Model file for the job. Use its own axes, mm. Coordinates: 2 decimals unless noted, no trailing zeros. Write each loop counter-clockwise with the first axis right and the second up, starting at its lowest first coordinate (ties: lowest second). Pieces come first, ordered by that corner, then holes. Notation, with made-up numbers: (3, 11) - (53, 11) arc R8 cw to (53, 20) - close; hole circle Ø11 at (7.25, 7.25). An arc over 180 degrees is marked (long way). Put each result on its own line as item: value. Start each with the question number.
1. Drill centre lines: L1, parallel to X at y = 29, z = 1.8; L2, parallel to X at y = 3, z = 4.05 (3 decimals); L3, parallel to Y at x = -29, z = 0.4. Where is each one in solid material? Low to high. Write a range as from..to.
2. Drop flat-ended pins along their axis: P1, Ø22, axis at x = 0, y = 32.78, coming from the +Z side; P2, Ø10, axis at x = 32.78, y = 0, coming from the +Z side; P3, Ø2, axis at x = -40, z = 3, coming from the +Y side; P4, Ø1, axis at x = -11.5, z = 1.5, coming from the -Y side (3 decimals). Give the stop position or say it passes through.
3. Saw through at A-A, the plane z = 3.2. Give the number of separate pieces and of enclosed holes in the cut face, plus the area to 3 significant figures.
4. Saw through at B-B, the plane x = 0. Write the cut outline in (y, z), plus the area to 3 significant figures.
```python
from build123d import *

# Parameters (mm, degrees)
F0_R     = 50
F0_R_2   = 8.5
F1_DEPTH = 5
F2_R     = 1


with BuildPart() as f1:
    # F0 (on Top) → F1 (new body)
    with BuildSketch(Plane.XY):
        Circle(F0_R)
        with Locations((-23.180378, -23.180378)):
            Circle(F0_R_2, mode=Mode.SUBTRACT)
        with Locations((0, -32.782005)):
            Circle(F0_R_2, mode=Mode.SUBTRACT)
        with Locations((23.180378, -23.180378)):
            Circle(F0_R_2, mode=Mode.SUBTRACT)
        with Locations((-32.782005, 0)):
            Circle(F0_R_2, mode=Mode.SUBTRACT)
        with Locations((-23.180378, 23.180378)):
            Circle(F0_R_2, mode=Mode.SUBTRACT)
        Polygon((3.381157, 3.683446), (4.880537, -1.086445), (1.499379, -4.769891), (-3.381157, -3.683446), (-4.880537, 1.086445), (-1.499379, 4.769891), align=None, mode=Mode.SUBTRACT)
        with Locations((23.180378, 23.180378)):
            Circle(F0_R_2, mode=Mode.SUBTRACT)
        with Locations((32.782005, 0)):
            Circle(F0_R_2, mode=Mode.SUBTRACT)
        with Locations((0, 32.782005)):
            Circle(F0_R_2, mode=Mode.SUBTRACT)
    extrude(amount=F1_DEPTH)

    # F2
    f2_edges = [f1.edges().sort_by_distance(p)[0] for p in [
        (-50, 0, 5),
        (-50, 0, 0),
    ]]
    fillet(f2_edges, radius=F2_R)


solid = f1.part
```
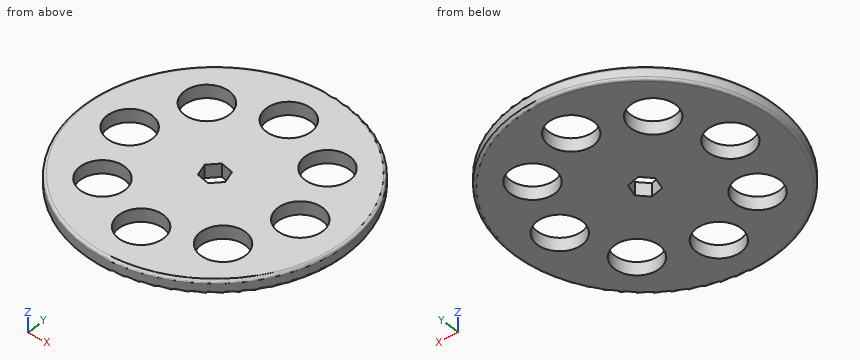
Final values:
1. L1: x = -40.73..-29.38, -16.99..-7.61, 7.61..16.99, 29.38..40.73
1. L2: x = -49.909..-40.735, -24.829..-3.124, 3.596..24.829, 40.735..49.909
1. L3: y = -40.49..-29.38, -16.99..-7.61, 7.61..16.99, 29.38..40.49
2. P1: stops at z = 5
2. P2: passes through
2. P3: stops at y = 31.29
2. P4: stops at y = -48.775
3. separate pieces: 1
3. enclosed holes: 9
3. area: 5,970 mm²
4. outline: (-50, 1) arc R1 ccw to (-49, 0) - (-41.28, 0) - (-41.28, 5) - (-49, 5) arc R1 ccw to (-50, 4) - close; (-24.28, 0) - (-4.44, 0) - (-4.44, 5) - (-24.28, 5) - close; (4.44, 0) - (24.28, 0) - (24.28, 5) - (4.44, 5) - close; (41.28, 0) - (49, 0) arc R1 ccw to (50, 1) - (50, 4) arc R1 ccw to (49, 5) - (41.28, 5) - close
4. area: 285 mm²
